from build123d import *

# Parameters (mm, degrees)
F0_R     = 22.225
F1_DEPTH = 11.2
F2_R     = 25.4
F2_R_2   = 22.225
F3_DEPTH = 2
F4_R     = 20.75
F5_DEPTH = 25
F6_R     = 1


with BuildPart() as f1:
    # F0 (on Top) → F1 (new body)
    with BuildSketch(Plane.XY):
        Circle(F0_R)
    extrude(amount=F1_DEPTH)

    # F2 (on face) → F3 (join)
    with BuildSketch(Plane.XY.offset(11.2)):
        Circle(F2_R)
        Circle(F2_R_2, mode=Mode.SUBTRACT)
    extrude(amount=-F3_DEPTH)

    # F4 (on face) → F5 (cut)
    with BuildSketch(Plane(origin=(0, 0, 0), x_dir=(1, 0, 0), z_dir=(0, 0, -1))):
        Circle(F4_R)
    extrude(amount=-F5_DEPTH, mode=Mode.SUBTRACT)

    # F6
    f6_edges = [f1.edges().sort_by_distance(p)[0] for p in [
        (-20.75, 0, 11.2),
    ]]
    fillet(f6_edges, radius=F6_R)


solid = f1.part
Design review of the part built by this model. Coordinates are the model's own, in mm. A direction names the side the tool comes from. Round coordinates to 2 decimals unless told otherwise and drop trailing zeros. Write each loop counter-clockwise with the first axis right and the second up, starting at its lowest first coordinate (ties: lowest second). Pieces come first, ordered by that corner, then holes.
Item 1: Draft analysis for pull direction X (two halves, no side actions). For faces 1 (the flat face through (19, 11, 11.2)), 2 (the cylindrical face through (-5.506, -24.796, 10.214)), 3 (the cylindrical face through (19.8, -6.2, 5)), state which applies: released by +X, released by -X, zero draft, split by the parting line, or undercut.
Item 2: Wall thickness on L1, parallel to Y at x = 0, z = 7.5 (3 decimals); L2, parallel to Y at x = 9, z = 10; L3, parallel to Z at x = 14, y = -19.5: over which ranges is each line inside the solid? List them lowest first.
Item 3: Consider section A-A on x = 0. Give the boundary of the cut face in (y, z) (3 decimals), and give its area (3 significant figures).
Item 4: Consider section C-C on z = 2.25. Give the boundary of the cut face in (x, y) (3 decimals), and give its area (3 significant figures).
Item 5: For pin 1 Ø3 at (x, z) = (14.5, 3) entering from -Y; pin 2 Ø4 at (x, z) = (-20.5, 4) entering from -Y; pin 3 Ø6 at (y, z) = (-16, 8) entering from +X, all flat-tipped, find the tip position at first contact; note any pin that passes through.
Item 6: For faces 4 (the flat face through (-7, -20, 0)), 5 (the cylindrical face through (21.199, 6.676, 4.536)), list the 3-axis set-ups (+Z, -Z, +X, -X, +Y, -Y) from which the entire face can be reached by the end or side of a thin tool; tool diameter is ignored.
Check values:
1. face 1: zero draft
1. face 2: split by the parting line
1. face 3: undercut
2. L1: y = -22.225 to -20.75, 20.75 to 22.225
2. L2: y = -23.75 to -18.7, 18.7 to 23.75
2. L3: z = 9.2 to 11.2
3. outline: (-25.4, 9.2) - (-22.225, 9.2) - (-22.225, 0) - (-20.75, 0) - (-20.75, 10.2) arc R1 ccw to (-21.75, 11.2) - (-25.4, 11.2) - close; (20.75, 0) - (22.225, 0) - (22.225, 9.2) - (25.4, 9.2) - (25.4, 11.2) - (21.75, 11.2) arc R1 ccw to (20.75, 10.2) - close
3. area: 45.3 mm2
4. outline: circle Ø44.45 at (0, 0); hole circle Ø41.5 at (0, 0)
4. area: 199 mm2
5. pin 1: stops at y = -18.03
5. pin 2: stops at y = -12.32
5. pin 3: stops at x = 21.67
6. face 4: -Z, +X, -X, +Y, -Y
6. face 5: -Z
